Autodesk Inventor part; units mm, degrees
ref_plane "YZ Plane" through (0, 0, 0) normal (1, 0, 0) x (0, 1, 0)
ref_plane "XZ Plane" through (0, 0, 0) normal (0, 1, 0) x (-1, 0, 0)
ref_plane "XY Plane" through (0, 0, 0) normal (0, 0, 1) x (1, 0, 0)
sketch "Sketch1" plane through (0, 0, 0) normal (0, 1, 0) x (-1, 0, 0)
  line L0 (-17.5, -17.5) -> (17.5, -17.5)
  line L1 (17.5, -17.5) -> (17.5, 17.5)
  line L2 (17.5, 17.5) -> (-17.5, 17.5)
  line L3 (-17.5, 17.5) -> (-17.5, -17.5)
  line L4 (-17.5, -17.5) -> (17.5, 17.5) construction
  line L5 (17.5, -17.5) -> (-17.5, 17.5) construction
  point P0 (0, 0)
  dimension "d0" = 35
  dimension "d1" = 35
extrude "Extrusion1" add sketch "Sketch1" along normal blind 3
sketch "Sketch2" plane through (0, 3, 0) normal (0, 1, 0) x (1, 0, 0)
  line L0 (-12.5, 5) -> (12.5, 5)
  line L1 (12.5, 5) -> (12.5, -5)
  line L2 (12.5, -5) -> (-12.5, -5)
  line L3 (-12.5, -5) -> (-12.5, 5)
  line L4 (-12.5, 5) -> (12.5, -5) construction
  line L5 (12.5, 5) -> (-12.5, -5) construction
  point P0 (0, 0)
  dimension "d4" = 25
  dimension "d5" = 10
extrude "Extrusion2" add sketch "Sketch2" along normal blind 50
sketch "Sketch3" plane through (-12.5, 3, 5) normal (0, 0, 1) x (1, 0, 0)
  line L0 (6.3, 38.5) -> (18.7, 38.5)
  line L1 (18.7, 38.5) -> (18.7, 15)
  line L2 (18.7, 15) -> (6.3, 15)
  line L3 (6.3, 15) -> (6.3, 38.5)
  line L4 (6.3, 38.5) -> (18.7, 15) construction
  line L5 (18.7, 38.5) -> (6.3, 15) construction
  line L6 (-5, 0) -> (30, 0)
  line L7 (0, 50) -> (25, 50)
  point P0 (12.5, -3)
  point P1 (12.5, 26.75)
  point P2 (12.5, 38.5)
  point P3 (12.5, 50)
  dimension "d8" = 12.4
  dimension "d9" = 23.5
  dimension "d10" = 15
fillet "Fillet1" radius 2 4 edges at (-12.5, 3, 0) (12.5, 3, 0) (0, 3, 5) (0, 3, -5)
extrude "Extrusion4" cut sketch "Sketch3" against normal through all
sketch "Sketch5" plane through (-12.5, 53, 5) normal (0, 0, 1) x (1, 0, 0)
  circle A0 centre (12.5, -9.35) radius 1.05
  line L0 (6.3, -11.5) -> (18.7, -11.5)
  line L1 (18.7, -11.5) -> (18.7, -35) construction
  line L2 (18.7, -23.25) -> (6.3, -23.25) construction
  circle A1 centre (12.5, -37.15) radius 1.05
  point P0 (12.5, -53)
  point P1 (12.5, -11.5)
  point P2 (12.5, -11.5)
  dimension "d18" = 2.1
  dimension "d19" = 2.15
extrude "Extrusion5" cut sketch "Sketch5" against normal blind 10
sketch "Sketch6" plane through (-6.2, 41.5, 5) normal (0, -1, 0) x (1, 0, 0)
  line L0 (12.4, 0) -> (12.4, -10)
  line L1 (0, 0) -> (0, -10)
  line L2 (0, 0) -> (12.4, 0)
  line L3 (12.4, -10) -> (0, -10)
  line L4 (8.05, -10) -> (4.35, -10)
  line L5 (4.35, -10) -> (4.35, 0)
  line L6 (4.35, 0) -> (8.05, 0)
  line L7 (8.05, 0) -> (8.05, -10)
  line L8 (8.05, -10) -> (4.35, 0) construction
  line L9 (4.35, -10) -> (8.05, 0) construction
  point P0 (6.2, -5)
  point P1 (6.2, -5)
  point P2 (6.2, -10)
  point P3 (6.2, -10)
  point P4 (8.05, -5)
  point P5 (12.4, -5)
  point P6 (8.05, 0)
  point P7 (4.35, 0)
  point P8 (4.35, -10)
  dimension "d22" = 3.7
  dimension "d23" = 10
extrude "Extrusion6" cut sketch "Sketch6" against normal blind 0.8 contours L7 L3 L5 L2
sketch "Sketch8" plane through (0, 0, 0) normal (0, -1, 0) x (1, 0, 0)
  line L0 (-17.5, 17.5) -> (17.5, 17.5)
  point P0 (0, 0)
  point P1 (0, 12.5)
  dimension "d41" = 5
hole "Hole2" at (0, 0, 12.5) direction (0, 1, 0) diameter 3.1 end through all
mirror "Mirror3" about plane through (0, 0, 0) normal (0, 0, 1) of "Hole2"
sketch "Sketch9" plane through (-6.2, 18, 5) normal (0, 1, 0) x (1, 0, 0)
  line L0 (4.35, 10) -> (4.35, 0)
  line L1 (8.05, 0) -> (8.05, 10)
  line L2 (4.35, 0) -> (8.05, 0)
  line L3 (8.05, 10) -> (4.35, 10)
  point P0 (6.2, 5)
extrude "Extrusion7" cut sketch "Sketch9" against normal blind 0.8
properties part number "base de motor"
Work out the finished part from the listing and answer in its coordinate system (mm). A direction names the side the tool comes from. Give positions to 0.01 mm unless a question says otherwise; leave off trailing zeros. Loops run counter-clockwise (first coordinate to the right, second up) from the corner with the lowest first, then second, coordinate; pieces in that order, holes last. Notation, with made-up numbers: (14, -40) - (33, -40) arc R34 ccw to (33, -3) - close; hole circle Ø4 at (37.5, -33.5). An arc over 180 degrees is marked (long way). Use CSV: the item, a comma, the result in double quotes. Start each with the question number.
(1) Find section C-C, the plane y = 40. Determine the outline of the cut face in (x, z), plus the area to 3 significant figures.
(2) Find section B-B, the plane z = -12.5. Determine the outline of the cut face in (x, y), plus the area to 3 significant figures.
(3) Determine the mould class of faces 1 (the face through (4, 41.5, 0)), 2 (the face through (12.5, 29, 0)), 3 (the face through (0, 0, 0)), 4 (the face through (0.2, 3.6, -5.57)) for opening direction Y: released by +Y, released by -Y, zero draft, split by the parting line, or undercut.
(4) Each of these flat-tipped pins is pushed along its axis until it touches: pin 1 (3 mm diameter, centred on x = 12, y = 22.5, fed in from -Z); pin 2 (3 mm diameter, centred on x = 0, z = -12.5, fed in from -Y); pin 3 (12 mm diameter, centred on y = 10, z = 1, fed in from +X); pin 4 (4 mm diameter, centred on x = 13, z = 13.5, fed in from +Y). Where does it stop, or does it pass through?
(5) Find section D-D, the plane x = 5. Determine the outline of the cut face in (y, z), plus the area to 3 significant figures.
(6) Find section A-A, the plane x = 0. Count the separate pieces of the cut face and the enclosed holes in it, plus the area to 3 significant figures.
(7) A tool of negligible diameter and unlimited length cuts with its end or side. For faces 5 (the face through (6.2, 30, 0)), 6 (the face through (13.07, 3.6, 0.1)), 7 (the face through (9, 29, 5)), from which of +Z, -Z, +X, -X, +Y, -Y can it reach the whole face along a straight path? Write none if from no direction.
(8) Find the intervals of material crossed by L1, parallel to Y at x = 0, z = -1.75; L2, parallel to Z at x = 0, y = 1; L3, parallel to Y at x = 5, z = -2, in increasing order.
Results found:
1,outline,"(-12.5, -5) - (-6.2, -5) - (-6.2, 5) - (-12.5, 5) - close; (6.2, -5) - (12.5, -5) - (12.5, 5) - (6.2, 5) - close"
1,area,"126 mm^2"
2,outline,"(-17.5, 0) - (-1.55, 0) - (-1.55, 3) - (-17.5, 3) - close; (1.55, 0) - (17.5, 0) - (17.5, 3) - (1.55, 3) - close"
2,area,"95.7 mm^2"
3,face 1,"undercut"
3,face 2,"zero draft"
3,face 3,"released by -Y"
3,face 4,"released by +Y"
4,pin 1,"z = -5"
4,pin 2,"through"
4,pin 3,"x = 12.77"
4,pin 4,"y = 3"
5,outline,"(0, -17.5) - (3, -17.5) - (3, -7) arc R2 cw to (5, -5) - (18, -5) - (18, 5) - (5, 5) arc R2 cw to (3, 7) - (3, 17.5) - (0, 17.5) - close; (41.5, -5) - (53, -5) - (53, 5) - (41.5, 5) - close"
5,area,"372 mm^2"
6,separate pieces,"6"
6,enclosed holes,"0"
6,area,"295 mm^2"
7,face 5,"+Z, -Z"
7,face 6,"+Z, -Z, +X, +Y"
7,face 7,"+Z, +X, -X, +Y"
8,L1,"0 to 14.8, 16.9 to 17.2, 42.3 to 42.6, 44.7 to 53"
8,L2,"-17.5 to -14.05, -10.95 to 10.95, 14.05 to 17.5"
8,L3,"0 to 18, 41.5 to 53"
